```python
from build123d import *

# Parameters (mm, degrees)
SKETCH009_W             = 84
SKETCH009_H             = 70
PAD002_DEPTH            = 2
SKETCH010_W             = 2
SKETCH010_H             = 7
PAD003_DEPTH            = 2
SKETCH012_W             = 8
SKETCH012_H             = 6.8
PAD004_DEPTH            = 4
SKETCH013_W             = 7
SKETCH013_H             = 6
PAD005_DEPTH            = 4
SKETCH011_W             = 8
SKETCH011_H             = 6.8
PAD006_DEPTH            = 4
SKETCH014_R             = 1.15
POCKET002_DEPTH         = 81.001
SKETCH016_R             = 1.15
POCKET003_DEPTH         = 8.501
SKETCH018_W             = 11.5
SKETCH018_H             = 11.5
POCKET004_DEPTH         = 5
POCKET005_DEPTH         = 5
POCKET006_DEPTH         = 5
SKETCH021_W             = 1
SKETCH021_H             = 7
PAD007_DEPTH            = 1
SKETCH022_W             = 9
SKETCH022_H             = 10
POCKET007_DEPTH         = 0.4
FILLET_R                = 3
BODY002_PITCH_ANGLE     = -90
BODY002_PLACEMENT_ANGLE = 90
PAD001_DEPTH            = 42
SKETCH007_W             = 11.5
SKETCH007_H             = 11.5
POCKET001_DEPTH         = 13
FILLET001_R             = 3
SKETCH025_W             = 6.5
SKETCH025_H             = 9
SKETCH025_W_2           = 9
SKETCH025_H_2           = 6.5
POCKET008_DEPTH         = 3.5


with BuildPart() as back:
    # Sketch009 → Pad002 (new body)
    with BuildSketch(Plane.XY):
        Rectangle(SKETCH009_W, SKETCH009_H)
    extrude(amount=PAD002_DEPTH)

    # Sketch010 (on Face6 of Pad002) → Pad003 (join)
    with BuildSketch(Plane.XY.offset(2)):
        with Locations((-38, -1)):
            Rectangle(SKETCH010_W, SKETCH010_H)
        Polygon((-21, 32), (39, 32), (39, -4), (37, -4), (37, 30), (-21, 30), align=None)
    extrude(amount=PAD003_DEPTH)

    # Sketch012 (on Face15 of Pad003) → Pad004 (join)
    with BuildSketch(Plane.YZ.offset(39)):
        with Locations((0, 5.4)):
            Rectangle(SKETCH012_W, SKETCH012_H)
    extrude(amount=-PAD004_DEPTH)

    # Sketch013 (on Face9 of Pad004) → Pad005 (join)
    with BuildSketch(Plane(origin=(-39, 0, 0), x_dir=(0, -1, 0), z_dir=(-1, 0, 0))):
        with Locations((1, 5)):
            Rectangle(SKETCH013_W, SKETCH013_H)
    extrude(amount=-PAD005_DEPTH)

    # Sketch011 (on Face16 of Pad003) → Pad006 (join)
    with BuildSketch(Plane(origin=(0, 32, 0), x_dir=(-1, 0, 0), z_dir=(0, 1, 0))):
        with Locations((-29, 5.4)):
            Rectangle(SKETCH011_W, SKETCH011_H)
        with Locations((14, 5.4)):
            Rectangle(SKETCH011_W, SKETCH011_H)
    extrude(amount=-PAD006_DEPTH)

    # Sketch014 (on Face44 of Pad006) → Pocket002 (cut, through all)
    with BuildSketch(Plane.YZ.offset(39)):
        with Locations((0, 5)):
            Circle(SKETCH014_R)
    extrude(amount=-POCKET002_DEPTH, mode=Mode.SUBTRACT)

    # Sketch016 → Pocket003 (cut, through all)
    with BuildSketch(Plane.XZ.offset(-26.5)):
        with Locations((-13, 5)):
            Circle(SKETCH016_R)
        with Locations((30, 5)):
            Circle(SKETCH016_R)
    extrude(amount=-POCKET003_DEPTH, mode=Mode.SUBTRACT)

    # Sketch018 (on Face5 of Pocket003) → Pocket004 (cut)
    with BuildSketch(Plane.XY.offset(2)):
        with Locations((0, 17.75)):
            Rectangle(SKETCH018_W, SKETCH018_H)
    extrude(amount=-POCKET004_DEPTH, mode=Mode.SUBTRACT)

    # Sketch019 (on Face31 of Pocket004) → Pocket005 (cut)
    with BuildSketch(Plane.XZ.offset(-28)):
        Polygon((29.125944, 9.042901), (33.258869, 4.499726), (33.258869, 9.042901), align=None)
    extrude(amount=-POCKET005_DEPTH, mode=Mode.SUBTRACT)

    # Sketch020 (on Face36 of Pocket005) → Pocket006 (cut)
    with BuildSketch(Plane(origin=(35, 0, 0), x_dir=(0, -1, 0), z_dir=(-1, 0, 0))):
        Polygon((2.77547, 8.938441), (6.386171, 3.079567), (6.386171, 8.938441), align=None)
    extrude(amount=-POCKET006_DEPTH, mode=Mode.SUBTRACT)

    # Sketch021 (on Face40 of Pocket006) → Pad007 (join)
    with BuildSketch(Plane.XY.offset(8)):
        with Locations((-38.5, -1)):
            Rectangle(SKETCH021_W, SKETCH021_H)
    extrude(amount=PAD007_DEPTH)

    # Sketch022 (on Face5 of Pocket005) → Pocket007 (cut)
    with BuildSketch(Plane.XY.offset(2)):
        with Locations((-30.3, 30)):
            Rectangle(SKETCH022_W, SKETCH022_H)
    extrude(amount=-POCKET007_DEPTH, mode=Mode.SUBTRACT)

    # Fillet
    fillet_edges = [back.edges().sort_by_distance(p)[0] for p in [
        (42, 35, 1),
        (-42, 35, 1),
    ]]
    fillet(fillet_edges, radius=FILLET_R)


with BuildPart() as back_1:
    # Body002 pitch: moved
    add(back.part.rotate(Axis((0, 0, 0), (0, 1, 0)), BODY002_PITCH_ANGLE))


with BuildPart() as back_2:
    # Body002 placement: moved
    add(back_1.part.rotate(Axis((0, 0, 0), (0, 0, 1)), BODY002_PLACEMENT_ANGLE))


with BuildPart() as curve:
    # Sketch006 → Pad001 (new body, symmetric)
    with BuildSketch(Plane.XY):
        with BuildLine():
            ThreePointArc((-35, 2.120911), (0.083645, 1.403594), (35, 4.9))
            Line((35, -0.1), (35, 4.9))
            Line((-35, -0.1), (35, -0.1))
            Line((-35, 2.120911), (-35, -0.1))
        make_face()
    extrude(amount=PAD001_DEPTH, both=True)

    # Sketch007 (on Face3 of Pad001) → Pocket001 (cut)
    with BuildSketch(Plane.XZ.offset(0.1)):
        with Locations((-17.75, 0)):
            Rectangle(SKETCH007_W, SKETCH007_H)
    extrude(amount=-POCKET001_DEPTH, mode=Mode.SUBTRACT)

    # Fillet001
    fillet001_edges = [curve.edges().sort_by_distance(p)[0] for p in [
        (-35, 1.010456, -42),
        (-35, 1.010456, 42),
    ]]
    fillet(fillet001_edges, radius=FILLET001_R)

    # Boolean: union Back
    add(back_2.part)

    # Sketch025 (on Face32 of Boolean) → Pocket008 (cut, symmetric)
    with BuildSketch(Plane.XZ.offset(2)):
        with Locations((-28.75, 0)):
            Rectangle(SKETCH025_W, SKETCH025_H)
        with Locations((-15.55, 13.625)):
            Rectangle(SKETCH025_W_2, SKETCH025_H_2)
        with Locations((-2.05, 0)):
            Rectangle(SKETCH025_W, SKETCH025_H)
        with Locations((-15.55, -13.625)):
            Rectangle(SKETCH025_W_2, SKETCH025_H_2)
    extrude(amount=POCKET008_DEPTH, both=True, mode=Mode.SUBTRACT)


solid = curve.part
```
Model file for the job. Use its own axes, mm. A direction names the side the tool comes from. Coordinates: 2 decimals unless noted, no trailing zeros. Order: outer loops, then holes, each group sorted by start corner. A loop starts at its lowest first (then second) coordinate and runs counter-clockwise, first axis right, second up. Notation, with made-up numbers: (50.25, -39) - (97.25, -39) arc R5 cw to (97.25, -35) - close; hole circle Ø3 at (26, 63). An arc over 180 degrees is marked (long way). Return JSON: item names as keys, results as strings. Group by question number.
1) Flat gauge pins, fed straight in: P1, Ø10, axis at x = -32, z = -29, coming from the -Y side; P2, Ø2, axis at x = 0.5, y = -4.5, coming from the -Z side; P3, Ø1, axis at x = -30.5, z = -20, coming from the -Y side; P4, Ø2, axis at x = 0, y = -5, coming from the -Z side. Where does each tip first touch, or does it go through?
2) Saw through at A-A, the plane y = -0.5. Write the cut outline in (x, z) (3 decimals).
3) Saw through at C-C, the plane x = 0. Write the cut outline in (y, z), plus the area to 3 significant figures.
4) Saw through at D-D, the plane z = -30. Write the cut outline in (x, y).
5) Mould opens along Z. For faces 1 (the flat face through (1.2, 0, 0)), 2 (the flat face through (-32, -3.8, 21.5)) say: released by +Z, released by -Z, zero draft, split by the parting line, or undercut.
6) Probe line 1 (Y direction, x = 0, z = -37); line 2 (X direction, y = -5, z = -38.15); line 3 (X direction, y = 1, z = 16). List the from-to ranges inside material, lowest first. Write a range as from..to.
7) Tool access for faces 3 (the flat face through (-31, -4, -7)), 4 (the flat face through (-4, -6, 37)), 5 (the flat face through (4, -4, 37)), 6 (the flat face through (4.5, -5, -37)), 7 (the flat face through (-11.05, 0, 14)): list every direction of +Z, -Z, +X, -X, +Y, -Y with a clear straight run to the whole face (end or side of a thin tool).
8) Saw through at B-B, the plane z = -13. Write the cut outline in (x, y).
Values found:
{
 "1": {"P1": "stops at y = -2", "P2": "stops at z = -39", "P3": "stops at y = -4", "P4": "passes through"},
 "2": {"outline": "(-35, -39) arc R3 ccw to (-32, -42) - (35, -42) - (35, 42) - (-32, 42) arc R3 ccw to (-35, 39) - close; hole (-32, -4.5) - (-25.5, -4.5) - (-25.5, 4.5) - (-32, 4.5) - close; hole (-23.5, -5.75) - (-12, -5.75) - (-12, 5.75) - (-23.5, 5.75) - close; hole (-20.05, -16.875) - (-11.05, -16.875) - (-11.05, -10.375) - (-20.05, -10.375) - close; hole (-20.05, 10.375) - (-11.05, 10.375) - (-11.05, 16.875) - (-20.05, 16.875) - close; hole (-5.3, -4.5) - (1.2, -4.5) - (1.2, 4.5) - (-5.3, 4.5) - close"},
 "3": {"outline": "(-9, -39) - (-6.15, -39) - (-6.15, -35) - (-8, -35) - (-8, -38) - (-9, -38) - close; (-8.8, 35) - (-6.15, 35) - (-6.15, 39) - (-8.8, 39) - close; (-3.85, -39) - (-2, -39) - (-2, -42) - (1.4, -42) - (1.4, -4.5) - (-2, -4.5) - (-2, -35) - (-3.85, -35) - close; (-3.85, 35) - (-2, 35) - (-2, 4.5) - (1.4, 4.5) - (1.4, 42) - (-2, 42) - (-2, 39) - (-3.85, 39) - close", "area": "289 mm²"},
 "4": {"outline": "(-35, -1.6) - (-25, -1.6) - (-25, -2) - (35, -2) - (35, 4.9) arc R292 cw to (-35, 2.12) - close"},
 "5": {"face 1": "undercut", "face 2": "zero draft"},
 "6": {"line 1": "y = -8..-6.15, -3.85..1.4", "line 2": "x = -2.5..-1.15, 1.15..4.5", "line 3": "x = -35..-20.05, -11.05..35"},
 "7": {"face 3": "+X, -X, -Y", "face 4": "-Z, -Y", "face 5": "+Z, +X, -Y", "face 6": "+Z, -Z, +X, -Y", "face 7": "+Y, -Y"},
 "8": {"outline": "(-35, -2) - (-32, -2) - (-32, -3.85) - (-28, -3.85) - (-28, -2) - (-20.05, -2) - (-20.05, 1.3) arc R292 cw to (-35, 2.12) - close; (-32, -8.8) - (-28, -8.8) - (-28, -6.15) - (-32, -6.15) - close; (-11.05, -2) - (35, -2) - (35, 4.9) arc R292 cw to (-11.05, 1.17) - close"}
}
